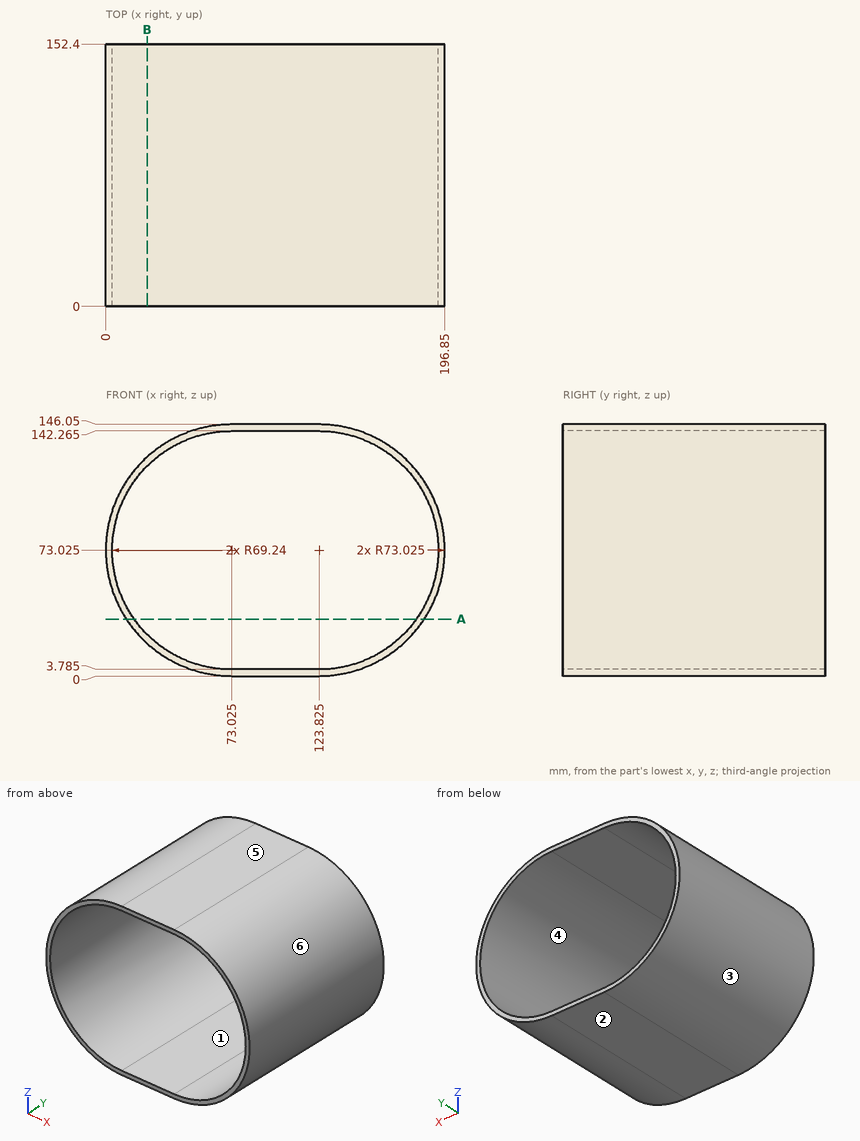
Part print with two shaded views. Sizes in mm from the minimum x, y, z corner. A direction names the side the tool comes from. Coordinates: 2 decimals unless noted, no trailing zeros. Loops run counter-clockwise (first coordinate to the right, second up) from the corner with the lowest first, then second, coordinate; pieces in that order, holes last. Notation, with made-up numbers: M 63.25,38 L 109.25,38 A17 ccw 109.25,64 Z; hole C 58.5,65.25 d10. An arc over 180 degrees is marked long. Use CSV: the item, a comma, the result in double quotes. Start each with the question number.
1. Tool access for the marked faces 1 and 2: list every direction of +Z, -Z, +X, -X, +Y, -Y with a clear straight run to the whole face (end or side of a thin tool).
2. Probe probe 1 along X at (y, z) = (85.5, 54); probe 2 along X at (y, z) = (9.5, 112) (1 decimal); probe 3 along Z at (x, y) = (41.5, 135.5) (1 decimal). List the from-to ranges inside material, lowest first. Write a range as [from, to].
3. Two-plate mould, pull along X, no slides. Class the marked faces 3, 4, 5 and 6: pulls with the +X half, pulls with the -X half, needs draft (parallel to the pull), parting line crosses it, or undercut.
4. Flat gauge pins, fed straight in: pin 1 (3 mm diameter, centred on y = 125, z = 20.5, fed in from +X) (1 decimal); pin 2 (3 mm diameter, centred on y = 68.5, z = 17, fed in from +X); pin 3 (1 mm diameter, centred on x = 20.5, y = 56, fed in from -Z). Where does each tip first touch, or does it go through?
5. Band-saw the part on A-A, the plane z = 33. List the corners of the cut face in (x, y) (1 decimal), then the cut area to 3 significant figures.
6. Band-saw the part on B-B, the plane x = 24. List the corners of the cut face in (y, z).
Entries:
1,face 1,"+Y, -Y"
1,face 2,"-Z, +X, -X, +Y, -Y"
2,probe 1,"x = [2.52, 6.45], [190.4, 194.33]"
2,probe 2,"x = [11.3, 15.8], [181.1, 185.6]"
2,probe 3,"z = [7.2, 11.4], [134.7, 138.9]"
3,face 3,"pulls with the -X half"
3,face 4,"undercut"
3,face 5,"needs draft"
3,face 6,"pulls with the +X half"
4,pin 1,"stops at x = 176.1"
4,pin 2,"stops at x = 172.4"
4,pin 3,"stops at z = 21.78"
5,outline,"M 11.9,0 L 16.5,0 L 16.5,152.4 L 11.9,152.4 Z; M 180.3,0 L 184.9,0 L 184.9,152.4 L 180.3,152.4 Z"
5,area,"1,400 mm2"
6,outline,"M 0,18.9 L 152.4,18.9 L 152.4,24.13 L 0,24.13 Z; M 0,121.92 L 152.4,121.92 L 152.4,127.15 L 0,127.15 Z"
